from build123d import *

# Parameters (mm, degrees)
CROQUIS1_W                = 40
CROQUIS1_H                = 50
SALIENTE_EXTRUIR1_DEPTH   = 15
CROQUIS2_R                = 1.75
CORTAR_EXTRUIR1_DEPTH     = 15
SIMETR_A2_COPY_1_SKETCH_R = 1.75
SIMETR_A2_COPY_1_DEPTH    = 15
CROQUIS3_W                = 6
CROQUIS3_H                = 6
CORTAR_EXTRUIR6_DEPTH     = 11
SIMETR_A4_COPY_1_SKETCH_W = 6
SIMETR_A4_COPY_1_SKETCH_H = 6
SIMETR_A4_COPY_1_DEPTH    = 11
CROQUIS4_W                = 35
CROQUIS4_H                = 10
CORTAR_EXTRUIR7_DEPTH     = 50.497474683
CROQUIS5_W                = 25
CROQUIS5_H                = 10
CORTAR_EXTRUIR8_DEPTH     = 56.901699437
REDONDEO1_R               = 5


with BuildPart() as part:
    # Croquis1 → Saliente-Extruir1 (new body)
    with BuildSketch(Plane(origin=(0, 0, 0), x_dir=(1, 0, 0), z_dir=(0, 1, 0))):
        Rectangle(CROQUIS1_W, CROQUIS1_H)
    extrude(amount=SALIENTE_EXTRUIR1_DEPTH)

    # Croquis2 → Cortar-Extruir1 (cut)
    with BuildSketch(Plane(origin=(0, 15, 0), x_dir=(1, 0, 0), z_dir=(0, 1, 0))):
        with Locations(Location((-17, 22, 0), (0, 0, 270))):
            Circle(CROQUIS2_R)
    cortar_extruir1 = extrude(amount=-CORTAR_EXTRUIR1_DEPTH, mode=Mode.SUBTRACT)

    # Simetría1: Cortar-Extruir1 across plane
    add(cortar_extruir1.mirror(Plane(origin=(0, 0, 0), x_dir=(0, 0, 1), z_dir=(1, 0, 0))), mode=Mode.SUBTRACT)

    # Simetría2: Cortar-Extruir1 across plane
    add(cortar_extruir1.mirror(Plane.XY), mode=Mode.SUBTRACT)

    # Simetría2 copy 1 sketch → Simetría2 copy 1 (cut)
    with BuildSketch(Plane(origin=(0, 15, 0), x_dir=(-1, 0, 0), z_dir=(0, 1, 0))):
        with Locations(Location((-17, 22, 0), (0, 0, 270))):
            Circle(SIMETR_A2_COPY_1_SKETCH_R)
    extrude(amount=-SIMETR_A2_COPY_1_DEPTH, mode=Mode.SUBTRACT)

    # Croquis3 → Cortar-Extruir6 (cut)
    with BuildSketch(Plane(origin=(0, 15, 0), x_dir=(1, 0, 0), z_dir=(0, 1, 0))):
        with Locations((-17, 22)):
            Rectangle(CROQUIS3_W, CROQUIS3_H)
    cortar_extruir6 = extrude(amount=-CORTAR_EXTRUIR6_DEPTH, mode=Mode.SUBTRACT)

    # Simetría3: Cortar-Extruir6 across plane
    add(cortar_extruir6.mirror(Plane(origin=(0, 0, 0), x_dir=(0, 0, 1), z_dir=(1, 0, 0))), mode=Mode.SUBTRACT)

    # Simetría4: Cortar-Extruir6 across plane
    add(cortar_extruir6.mirror(Plane.XY), mode=Mode.SUBTRACT)

    # Simetría4 copy 1 sketch → Simetría4 copy 1 (cut)
    with BuildSketch(Plane(origin=(0, 15, 0), x_dir=(-1, 0, 0), z_dir=(0, 1, 0))):
        with Locations((-17, 22)):
            Rectangle(SIMETR_A4_COPY_1_SKETCH_W, SIMETR_A4_COPY_1_SKETCH_H)
    extrude(amount=-SIMETR_A4_COPY_1_DEPTH, mode=Mode.SUBTRACT)

    # Croquis4 → Cortar-Extruir7 (cut, through all)
    with BuildSketch(Plane.ZY.offset(20)):
        with Locations((0, 5)):
            Rectangle(CROQUIS4_W, CROQUIS4_H)
    extrude(amount=-CORTAR_EXTRUIR7_DEPTH, mode=Mode.SUBTRACT)

    # Croquis5 → Cortar-Extruir8 (cut, through all)
    with BuildSketch(Plane.XY.offset(25)):
        with Locations((0, 5)):
            Rectangle(CROQUIS5_W, CROQUIS5_H)
    extrude(amount=-CORTAR_EXTRUIR8_DEPTH, mode=Mode.SUBTRACT)

    # Redondeo1
    redondeo1_edges = [part.edges().sort_by_distance(p)[0] for p in [
        (12.5, 5, 17.5),
        (-12.5, 5, 17.5),
        (-12.5, 5, -17.5),
        (12.5, 5, -17.5),
    ]]
    fillet(redondeo1_edges, radius=REDONDEO1_R)


solid = part.part
The model under review builds one solid part; all positions refer to its coordinate system, in mm. A direction names the side the tool comes from. Coordinates: 2 decimals unless noted, no trailing zeros. Write each loop counter-clockwise with the first axis right and the second up, starting at its lowest first coordinate (ties: lowest second). Pieces come first, ordered by that corner, then holes. Notation, with made-up numbers: (-2.5, 70.25) - (52.5, 70.25) arc R25 ccw to (52.5, 95.25) - close; hole circle Ø1 at (-31, 35). An arc over 180 degrees is marked (long way). Answer as a JSON object with one key per item and string values. Group by question number.
1. To check wall thickness, follow probe 1 along Z at (x, y) = (18.5, 1); probe 2 along X at (y, z) = (2.75, -22); probe 3 along Z at (x, y) = (17, 11). State the ranges of each line that lie inside material, in increasing order.
2. Add section B-B (x = -5.5). Give the boundary of the cut face in (y, z), plus the area to 3 significant figures.
3. Clearance check with flat-ended pins moving along their axes: pin 1 Ø6.5 at (y, z) = (10.5, 22) entering from -X; pin 2 Ø5 at (x, z) = (-18, 22.5) entering from +Y; pin 3 Ø3 at (y, z) = (6, -24) entering from -X; pin 4 Ø2 at (y, z) = (5.5, 24) entering from +X. State where each tip first meets the part, or that it passes through.
4. Machinability: for faces 4 (the face through (-12.5, 5, 24)), 5 (the face through (-18.4, 4, 20.7)), 6 (the face through (19, 5, 17.5)), which of the approach directions +Z, -Z, +X, -X, +Y, -Y give a long, thin tool a straight path to every point of the face, cutting with its end or side? Answer none if there is none.
5. Add section A-A (z = 7). Give the boundary of the cut face in (x, y).
6. Mouldability with a two-part tool opening along Z and no side actions: class faces 1 (the face through (-14, 10, -22)), 2 (the face through (14.587, 5.07, -18.436)), 3 (the face through (0, 11, 25)) as pulls with the +Z half, pulls with the -Z half, needs draft (parallel to the pull), parting line crosses it, or undercut.
Findings:
{
 "1": {"probe 1": "-25 to -22.9, -21.1 to -17.5, 17.5 to 21.1, 22.9 to 25", "probe 2": "-20 to -18.75, -15.25 to -12.53, 12.53 to 15.25, 18.75 to 20", "probe 3": "-19 to 19"},
 "2": {"outline": "(10, -25) - (15, -25) - (15, 25) - (10, 25) - close", "area": "250 mm²"},
 "3": {"pin 1": "x = -20", "pin 2": "y = 4", "pin 3": "x = -14", "pin 4": "x = 14"},
 "4": {"face 4": "+Z, -Z, -Y", "face 5": "+Z, -X, +Y", "face 6": "+X, -X, -Y"},
 "5": {"outline": "(-20, 10) - (20, 10) - (20, 15) - (-20, 15) - close"},
 "6": {"face 1": "needs draft", "face 2": "undercut", "face 3": "pulls with the +Z half"}
}
